```python
from build123d import *

# Parameters (mm, degrees)
RESSALTO_EXTRUS_O1_DEPTH  = 16
ESBO_O2_W                 = 2.8
ESBO_O2_H                 = 2.8
CORTE_EXTRUS_O1_DEPTH     = 54.103672189
ESBO_O4_W                 = 2.8
ESBO_O4_H                 = 2.8
CORTE_EXTRUS_O2_DEPTH     = 31.186917696
CORPO_MOVER_COPIAR1_ANGLE = 90
ESBO_O6_W                 = 30
ESBO_O6_H                 = 16
CORTE_EXTRUS_O3_DEPTH     = 29.861739379
ESBO_O7_W                 = 25.221413321
ESBO_O7_H                 = 12.57615678
RESSALTO_EXTRUS_O2_DEPTH  = 2.5
ESBO_O8_W                 = 2.8
ESBO_O8_H                 = 2.8
CORTE_EXTRUS_O4_DEPTH     = 29.271009886


with BuildPart() as part:
    # Esboço1 → Ressalto-extrusão1 (new body)
    with BuildSketch(Plane.XY):
        Polygon((-25, 0), (25, 0), (25, 8), (23.5, 8), (18, 2.5), (-18, 2.5), (-23.5, 8), (-25, 8), align=None)
    extrude(amount=RESSALTO_EXTRUS_O1_DEPTH)

    # Esboço2 → Corte-extrusão1 (cut, through all)
    with BuildSketch(Plane(origin=(25, 0, 0), x_dir=(0, 0, -1), z_dir=(1, 0, 0))):
        with Locations((-4, 4)):
            Rectangle(ESBO_O2_W, ESBO_O2_H)
        with Locations((-12, 4)):
            Rectangle(ESBO_O2_W, ESBO_O2_H)
    extrude(amount=-CORTE_EXTRUS_O1_DEPTH, mode=Mode.SUBTRACT)

    # Esboço4 → Corte-extrusão2 (cut, through all)
    with BuildSketch(Plane(origin=(0, 2.5, 0), x_dir=(1, 0, 0), z_dir=(0, 1, 0))):
        with Locations((-16, -4)):
            Rectangle(ESBO_O4_W, ESBO_O4_H)
        with Locations((-8, -4)):
            Rectangle(ESBO_O4_W, ESBO_O4_H)
        with Locations((0, -4)):
            Rectangle(ESBO_O4_W, ESBO_O4_H)
        with Locations((8, -4)):
            Rectangle(ESBO_O4_W, ESBO_O4_H)
        with Locations((16, -4)):
            Rectangle(ESBO_O4_W, ESBO_O4_H)
        with Locations((-8, -12)):
            Rectangle(ESBO_O4_W, ESBO_O4_H)
        with Locations((0, -12)):
            Rectangle(ESBO_O4_W, ESBO_O4_H)
        with Locations((8, -12)):
            Rectangle(ESBO_O4_W, ESBO_O4_H)
        with Locations((16, -12)):
            Rectangle(ESBO_O4_W, ESBO_O4_H)
        with Locations((-16, -12)):
            Rectangle(ESBO_O4_W, ESBO_O4_H)
    extrude(amount=-CORTE_EXTRUS_O2_DEPTH, mode=Mode.SUBTRACT)


with BuildPart() as part_1:
    # Corpo-Mover/Copiar1: moved
    add(part.part.rotate(Axis((0, 4, 8), (1, 0, 0)), CORPO_MOVER_COPIAR1_ANGLE))

    # Esboço6 → Corte-extrusão3 (cut, through all)
    with BuildSketch(Plane(origin=(0, 0, 4), x_dir=(-1, 0, 0), z_dir=(0, 0, -1))):
        with Locations((-10, 4)):
            Rectangle(ESBO_O6_W, ESBO_O6_H)
    extrude(amount=-CORTE_EXTRUS_O3_DEPTH, mode=Mode.SUBTRACT)

    # Espelhar3: part across plane


with BuildPart() as part_2:
    add(part_1.part)
    add(part_1.part.mirror(Plane(origin=(-5, -4, 12), x_dir=(0, 0, 1), z_dir=(-1, 0, 0))))

    # Esboço7 → Ressalto-extrusão2 (add, through all)
    with BuildSketch(Plane.XY.offset(6.5)):
        with Locations((-4.971284079, 3.626460754)):
            Rectangle(ESBO_O7_W, ESBO_O7_H)
    extrude(amount=-RESSALTO_EXTRUS_O2_DEPTH)

    # Esboço8 → Corte-extrusão4 (cut, through all)
    with BuildSketch(Plane.XY.offset(6.5)):
        with Locations((-5, 8)):
            Rectangle(ESBO_O8_W, ESBO_O8_H)
        with Locations((-13, 8)):
            Rectangle(ESBO_O8_W, ESBO_O8_H)
        with Locations((3, 8)):
            Rectangle(ESBO_O8_W, ESBO_O8_H)
        with Locations((-5, 0)):
            Rectangle(ESBO_O8_W, ESBO_O8_H)
        with Locations((3, 0)):
            Rectangle(ESBO_O8_W, ESBO_O8_H)
        with Locations((-13, 0)):
            Rectangle(ESBO_O8_W, ESBO_O8_H)
    extrude(amount=-CORTE_EXTRUS_O4_DEPTH, mode=Mode.SUBTRACT)


solid = part_2.part
```
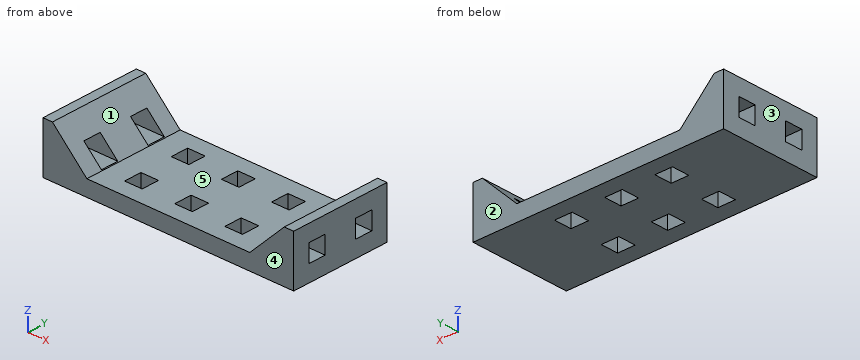
Design review of the part built by this model. Coordinates are the model's own, in mm. Face numbers are marked on the shaded views. A direction names the side the tool comes from. Coordinates: 2 decimals unless noted, no trailing zeros. Write each loop counter-clockwise with the first axis right and the second up, starting at its lowest first coordinate (ties: lowest second). Pieces come first, ordered by that corner, then holes.
1) Add section A-A (z = 7). Write out the cut boundary in (x, y).
2) Add section C-C (z = 10.75). Write out the cut boundary in (x, y).
3) Add section D-D (y = -0.5). Write out the cut boundary in (x, z), plus the area to 4 significant figures.
4) Machinability: for the marked faces 1 and 2, which of the approach directions +Z, -Z, +X, -X, +Y, -Y give a long, thin tool a straight path to every point of the face, cutting with its end or side? Answer none if there is none.
5) To check wall thickness, follow L1, parallel to X at y = 7, z = 6; L2, parallel to Z at x = 13.5, y = 8.25; L3, parallel to Z at x = -3, y = 9.25. State the ranges of each line that lie inside material, in increasing order.
6) Mouldability with a two-part tool opening along X and no side actions: class the marked faces 3, 4 and 5 as +X half, -X half, draft (parallel to the pull), parting line (faces both ways), or undercut.
7) Add section B-B (x = -5). Write out the cut boundary in (y, z), plus the area to 3 significant figures.
8) Insertion check: pin 1 (3 mm diameter, centred on x = 3.5, y = 2, fed in from +Z). The pin has a flat end and moves straight along its axis. Give the tip position at first contact, or say it passes through.
Check result:
1. outline: (-25, -4) - (-18.5, -4) - (-18.5, -1.4) - (-25, -1.4) - close; (-25, 1.4) - (-18.5, 1.4) - (-18.5, 6.6) - (-25, 6.6) - close; (-25, 9.4) - (-18.5, 9.4) - (-18.5, 12) - (-25, 12) - close; (8.5, -4) - (15, -4) - (15, -1.4) - (8.5, -1.4) - close; (8.5, 1.4) - (15, 1.4) - (15, 6.6) - (8.5, 6.6) - close; (8.5, 9.4) - (15, 9.4) - (15, 12) - (8.5, 12) - close
2. outline: (-25, -4) - (-22.25, -4) - (-22.25, 12) - (-25, 12) - close; (12.25, -4) - (15, -4) - (15, 12) - (12.25, 12) - close
3. outline: (-25, 4) - (-14.4, 4) - (-14.4, 6.5) - (-18, 6.5) - (-18.1, 6.6) - (-25, 6.6) - close; (-25, 9.4) - (-20.9, 9.4) - (-23.5, 12) - (-25, 12) - close; (-11.6, 4) - (-6.4, 4) - (-6.4, 6.5) - (-11.6, 6.5) - close; (-3.6, 4) - (1.6, 4) - (1.6, 6.5) - (-3.6, 6.5) - close; (4.4, 4) - (15, 4) - (15, 6.6) - (8.1, 6.6) - (8, 6.5) - (4.4, 6.5) - close; (10.9, 9.4) - (15, 9.4) - (15, 12) - (13.5, 12) - close
3. area: 94.95 mm2
4. face 1: +Z, +Y, -Y
4. face 2: +Z, -Z, +X, -X, +Y
5. L1: x = -25 to -14.4, -11.6 to -6.4, -3.6 to 1.6, 4.4 to 15
5. L2: z = 4 to 6.6, 9.4 to 12
5. L3: z = 4 to 6.5
6. face 3: -X half
6. face 4: draft
6. face 5: undercut
7. outline: (-4, 4) - (-1.4, 4) - (-1.4, 6.5) - (-4, 6.5) - close; (1.4, 4) - (6.6, 4) - (6.6, 6.5) - (1.4, 6.5) - close; (9.4, 4) - (12, 4) - (12, 6.5) - (9.4, 6.5) - close
7. area: 26.0 mm2
8. pin 1: stops at z = 6.5
